```python
from build123d import *

# Parameters (mm, degrees)
F0_R     = 2.5
F1_DEPTH = 2
F2_R     = 31.49999


# Not quite as in the source:
# - a fillet or chamfer is up to 0.001 mm smaller than in the source, because OpenCascade refuses the exact size


with BuildPart() as f1:
    # F0 (on Front) → F1 (new body)
    with BuildSketch(Plane.XZ):
        Polygon((-61.5, 0), (0, 0), (61.5, 0), (61.5, 370), (31.5, 370), (31.5, 290), (5.5, 290), (-5.5, 290), (-31.5, 290), (-31.5, 370), (-61.5, 370), align=None)
        with Locations((-52.6, 100)):
            Circle(F0_R, mode=Mode.SUBTRACT)
        with Locations((52.6, 100)):
            Circle(F0_R, mode=Mode.SUBTRACT)
        with Locations((-52.6, 270)):
            Circle(F0_R, mode=Mode.SUBTRACT)
        with Locations((52.6, 270)):
            Circle(F0_R, mode=Mode.SUBTRACT)
    extrude(amount=F1_DEPTH)

    # F2 (radius 31.5 in the source; OpenCascade refuses exactly that, so slightly less here)
    f2_edges = [f1.edges().sort_by_distance(p)[0] for p in [
        (-31.5, -1, 290),
        (31.5, -1, 290),
    ]]
    fillet(f2_edges, radius=F2_R)


solid = f1.part
```
CAD build for the part. Positions are in the model's coordinates, mm. A direction names the side the tool comes from. Give positions to 0.01 mm unless a question says otherwise; leave off trailing zeros. Order: outer loops, then holes, each group sorted by start corner. A loop starts at its lowest first (then second) coordinate and runs counter-clockwise, first axis right, second up. Notation, with made-up numbers: M 21,24 L 41,24 A17 ccw 41,31 Z; hole C -21,42.5 d5. An arc over 180 degrees is marked long. Put each result on its own line as item: value. Start each with the question number.
(1) Which spindle directions (+Z, -Z, +X, -X, +Y, -Y) get a long thin tool onto all of the face, cutting with end or side? Do faces 1 (the cylindrical face through (-22.517, -1.014, 299.472)), 2 (the flat face through (-1, 0, 146)). Say none if no direction does.
(2) Saw through at B-B, the plane x = -5. Write the cut outline in (y, z), then the cut area to 3 significant figures.
(3) Mould opens along X. For faces 3 (the cylindrical face through (22.517, -1.014, 299.472)), 4 (the flat face through (-1, -2, 146)) say: +X half, -X half, draft (parallel to the pull), parting line (faces both ways), or undercut.
(4) Drill centre lines: line 1 along X through (y, z) = (-1.05, 270); line 2 along Z through (x, y) = (-52.6, -1.5); line 3 along X through (y, z) = (-1.75, 328). Where is each one in solid material? Low to high.
(5) Saw through at A-A, the plane y = -0.9. Give the number of separate pieces and of enclosed holes in the cut face, then the cut area to 3 significant figures.
Check result:
1. face 1: +Z, +Y, -Y
1. face 2: +Z, -Z, +X, -X, +Y
2. outline: M -2,0 L 0,0 L 0,290.4 L -2,290.4 Z
2. area: 581 mm2
3. face 3: undercut
3. face 4: draft
4. line 1: x = -61.5 to -55.1, -50.1 to 50.1, 55.1 to 61.5
4. line 2: z = 0 to 97.5, 102.5 to 267.5, 272.5 to 370
4. line 3: x = -61.5 to -31.5, 31.5 to 61.5
5. separate pieces: 1
5. enclosed holes: 4
5. area: 40,800 mm2
